Can you work these out from the model? Positions are in its coordinate system, mm. A direction names the side the tool comes from. Round coordinates to 2 decimals unless told otherwise and drop trailing zeros. Loops run counter-clockwise (first coordinate to the right, second up) from the corner with the lowest first, then second, coordinate; pieces in that order, holes last. Notation, with made-up numbers: (6.5, -39.75) -> (22.5, -39.75) arc R8 ccw to (22.5, -34.75) -> close; hole circle Ø5 at (64.5, 8). An arc over 180 degrees is marked (long way). Answer as a JSON object with one key per item and string values.
```python
from build123d import *

# Parameters (mm, degrees)
SKETCH1_W           = 45.23
SKETCH1_H           = 20.45
BOSS_EXTRUDE1_DEPTH = 1.6
SKETCH2_R           = 7.92
BOSS_EXTRUDE2_DEPTH = 12.2
BOSS_EXTRUDE3_DEPTH = 3.3
SKETCH4_W           = 4
SKETCH4_H           = 10.1
SKETCH4_W_2         = 8.68
SKETCH4_H_2         = 5.15
SKETCH4_W_3         = 10.3
SKETCH4_H_3         = 2.53
BOSS_EXTRUDE4_DEPTH = 1
SKETCH5_W           = 10.3
SKETCH5_H           = 2.53
BOSS_EXTRUDE5_DEPTH = 3.5
SKETCH6_R           = 0.25
BOSS_EXTRUDE6_DEPTH = 6.3
FILLET1_R           = 0.5
FILLET2_R           = 0.5
FILLET3_R           = 0.2
FILLET4_R           = 0.5
SKETCH7_R           = 0.55
CUT_EXTRUDE1_DEPTH  = 6.3


with BuildPart() as part:
    # Sketch1 → Boss-Extrude1 (new body)
    with BuildSketch(Plane(origin=(0, 0, 0), x_dir=(1, 0, 0), z_dir=(0, 1, 0))):
        with Locations((-22.615, 10.225)):
            Rectangle(SKETCH1_W, SKETCH1_H)
    extrude(amount=BOSS_EXTRUDE1_DEPTH)

    # Sketch2 → Boss-Extrude2 (add)
    with BuildSketch(Plane(origin=(0, 1.6, 0), x_dir=(1, 0, 0), z_dir=(0, 1, 0))):
        with Locations(Location((-35.515, 10.225, 0), (0, 0, 270))):
            Circle(SKETCH2_R)
        with Locations(Location((-9.715, 10.225, 0), (0, 0, 270))):
            Circle(SKETCH2_R)
    extrude(amount=BOSS_EXTRUDE2_DEPTH)

    # Sketch3 → Boss-Extrude3 (add)
    with BuildSketch(Plane(origin=(0, 1.6, 0), x_dir=(1, 0, 0), z_dir=(0, 1, 0))):
        with BuildLine():
            Line((-25.77, 19.5), (-19.46, 19.5))
            ThreePointArc((-19.46, 19.5), (-17.74, 17.78), (-19.46, 16.06))
            Line((-19.46, 16.06), (-25.77, 16.06))
            ThreePointArc((-25.77, 16.06), (-27.49, 17.78), (-25.77, 19.5))
        make_face()
    extrude(amount=BOSS_EXTRUDE3_DEPTH)

    # Sketch4 → Boss-Extrude4 (add)
    with BuildSketch(Plane.XZ):
        with Locations((-40.73, -10.225)):
            Rectangle(SKETCH4_W, SKETCH4_H)
        with Locations((-22.615, -10.225)):
            Rectangle(SKETCH4_W_2, SKETCH4_H_2)
        with Locations((-4.34, -10.225)):
            Rectangle(SKETCH4_W_2, SKETCH4_H_2)
        with Locations((-22.615, -1.465)):
            Rectangle(SKETCH4_W_3, SKETCH4_H_3)
    extrude(amount=BOSS_EXTRUDE4_DEPTH)

    # Sketch5 → Boss-Extrude5 (add)
    with BuildSketch(Plane.XZ.offset(1)):
        with Locations((-22.615, -1.465)):
            Rectangle(SKETCH5_W, SKETCH5_H)
    extrude(amount=BOSS_EXTRUDE5_DEPTH)

    # Sketch6 → Boss-Extrude6 (add)
    with BuildSketch(Plane.XY.offset(-0.2)):
        with Locations((-21.334010663, -4.5)):
            Circle(SKETCH6_R)
        with Locations((-18.759010663, -4.5)):
            Circle(SKETCH6_R)
        with Locations(Location((-23.895989337, -4.5, 0), (0, 0, 180))):
            Circle(SKETCH6_R)
        with Locations(Location((-26.470989337, -4.5, 0), (0, 0, 180))):
            Circle(SKETCH6_R)
    extrude(amount=BOSS_EXTRUDE6_DEPTH)

    # Fillet1
    # the kernel refuses this fillet: 0.5 mm, written as the material it adds along each edge
    with BuildSketch(Plane(origin=(-24.970989337, -4.5, -0.2), x_dir=(0, 0, -1), z_dir=(-1, 0, 0))) as fillet1_piece_1_section:
        with BuildLine():
            CenterArc((FILLET1_R, FILLET1_R), FILLET1_R, 180, 90)
            Line((0, FILLET1_R), (0, 0))
            Line((0, 0), (FILLET1_R, 0))
        make_face()
    fillet1_piece_1 = extrude(amount=3, mode=Mode.PRIVATE)
    fillet1_piece_1 = fillet1_piece_1 & Plane(origin=(-26.470989337, -4.5, -0.330121351), x_dir=(-1, 0, 0), z_dir=(0, 0, -1)) * Cylinder(0.25, 8, mode=Mode.PRIVATE)
    add(fillet1_piece_1)
    with BuildSketch(Plane(origin=(-22.395989337, -4.5, -0.2), x_dir=(0, 0, -1), z_dir=(-1, 0, 0))) as fillet1_piece_2_section:
        with BuildLine():
            CenterArc((FILLET1_R, FILLET1_R), FILLET1_R, 180, 90)
            Line((0, FILLET1_R), (0, 0))
            Line((0, 0), (FILLET1_R, 0))
        make_face()
    fillet1_piece_2 = extrude(amount=3, mode=Mode.PRIVATE)
    fillet1_piece_2 = fillet1_piece_2 & Plane(origin=(-23.895989337, -4.5, -0.330121351), x_dir=(-1, 0, 0), z_dir=(0, 0, -1)) * Cylinder(0.25, 8, mode=Mode.PRIVATE)
    add(fillet1_piece_2)
    with BuildSketch(Plane(origin=(-19.834010663, -4.5, -0.2), x_dir=(0, 0, -1), z_dir=(-1, 0, 0))) as fillet1_piece_3_section:
        with BuildLine():
            CenterArc((FILLET1_R, FILLET1_R), FILLET1_R, 180, 90)
            Line((0, FILLET1_R), (0, 0))
            Line((0, 0), (FILLET1_R, 0))
        make_face()
    fillet1_piece_3 = extrude(amount=3, mode=Mode.PRIVATE)
    fillet1_piece_3 = fillet1_piece_3 & Plane(origin=(-21.334010663, -4.5, -0.330121598), x_dir=(1, 0, 0), z_dir=(0, 0, -1)) * Cylinder(0.25, 8, mode=Mode.PRIVATE)
    add(fillet1_piece_3)
    with BuildSketch(Plane(origin=(-17.259010663, -4.5, -0.2), x_dir=(0, 0, -1), z_dir=(-1, 0, 0))) as fillet1_piece_4_section:
        with BuildLine():
            CenterArc((FILLET1_R, FILLET1_R), FILLET1_R, 180, 90)
            Line((0, FILLET1_R), (0, 0))
            Line((0, 0), (FILLET1_R, 0))
        make_face()
    fillet1_piece_4 = extrude(amount=3, mode=Mode.PRIVATE)
    fillet1_piece_4 = fillet1_piece_4 & Plane(origin=(-18.759010663, -4.5, -0.330121598), x_dir=(1, 0, 0), z_dir=(0, 0, -1)) * Cylinder(0.25, 8, mode=Mode.PRIVATE)
    add(fillet1_piece_4)

    # Fillet2
    fillet2_edges = [part.edges().sort_by_distance(p)[0] for p in [
        (-35.515, 13.8, -18.145),
        (-9.715, 13.8, -18.145),
    ]]
    fillet(fillet2_edges, radius=FILLET2_R)

    # Fillet3
    fillet3_edges = [part.edges().sort_by_distance(p)[0] for p in [
        (-27.49, 4.9, -17.78),
        (-22.615, 4.9, -16.06),
        (-17.74, 4.9, -17.78),
        (-22.615, 4.9, -19.5),
    ]]
    fillet(fillet3_edges, radius=FILLET3_R)

    # Fillet4
    fillet4_edges = [part.edges().sort_by_distance(p)[0] for p in [
        (-27.49, 1.6, -17.78),
        (-22.615, 1.6, -16.06),
        (-17.74, 1.6, -17.78),
        (-22.615, 1.6, -19.5),
    ]]
    fillet(fillet4_edges, radius=FILLET4_R)

    # Sketch7 → Cut-Extrude1 (cut)
    with BuildSketch(Plane(origin=(0, 1.6, 0), x_dir=(1, 0, 0), z_dir=(0, 1, 0))):
        with Locations(Location((-44.48, 19.7, 0), (0, 0, 270))):
            Circle(SKETCH7_R)
        with Locations(Location((-44.48, 0.75, 0), (0, 0, 270))):
            Circle(SKETCH7_R)
        with Locations(Location((-0.75, 0.75, 0), (0, 0, 270))):
            Circle(SKETCH7_R)
        with Locations(Location((-0.75, 19.7, 0), (0, 0, 270))):
            Circle(SKETCH7_R)
    extrude(amount=-CUT_EXTRUDE1_DEPTH, mode=Mode.SUBTRACT)


solid = part.part
```
Q1. I want a section at D-D, the plane x = -0.75. Write out the boundary of the cut face in (y, z).
Determined:
{"outline": "(-1, -12.8) -> (0, -12.8) -> (0, -19.15) -> (1.6, -19.15) -> (1.6, -1.3) -> (0, -1.3) -> (0, -7.65) -> (-1, -7.65) -> close; (0, -20.45) -> (1.6, -20.45) -> (1.6, -20.25) -> (0, -20.25) -> close; (0, -0.2) -> (1.6, -0.2) -> (1.6, 0) -> (0, 0) -> close"}
Q2. On a 3-axis mill with a long thin cutter (end or side, diameter ignored), from which of +Z, -Z, +X, -X, +Y, -Y can I reach the whole of each face in a straight line? I mean faces 4 (the flat face through (-22.7, -0.5, -7.65)), 5 (the flat face through (-23, -1, -10)), 6 (the cylindrical face through (-17.74, 3.38, -17.82)), 7 (the flat face through (-4.4, -0.5, -7.65)). Say none if no direction works.
Determined:
{"face 4": "+X, -Y", "face 5": "-Z, +X, -X, -Y", "face 6": "+Y", "face 7": "+Z, +X, -Y"}
Q3. I'm going to push flat-ended pins straight in: pin 1 (0.7 mm diameter, centred on x = -0.75, z = -19.7, fed in from +Y); pin 2 (10 mm diameter, centred on x = -12.5, z = -13.5, fed in from -Y); pin 3 (10 mm diameter, centred on x = -18, y = 6, fed in from +Z); pin 4 (1.4 mm diameter, centred on x = -0.75, z = -0.75, fed in from +Y). Where does each tip first touch, or does it pass through?
Determined:
{"pin 1": "through", "pin 2": "y = -1", "pin 3": "z = 0", "pin 4": "y = 1.6"}
Q4. We'd pull the mould along X, two halves only. Please class faces 1 (the flat face through (-27.765, -2, -1)), 2 (the flat face through (-23, -2, -2.73)), 3 (the cylindrical face through (-44.97, 0.81, -0.5)): pulls with the +X half, pulls with the -X half, needs draft (parallel to the pull), parting line crosses it, or undercut.
Determined:
{"face 1": "pulls with the -X half", "face 2": "needs draft", "face 3": "undercut"}
Q5. If I drill on L1, parallel to X at y = 1, z = -0.75; L2, parallel to Y at x = -38, z = -17; L3, parallel to X at y = 9, z = -11.5, over which ranges is the centre line in solid material (lowest first)? Write a range as [from, to].
Determined:
{"L1": "[-45.23, -45.03], [-43.93, -1.3], [-0.2, 0]", "L2": "[0, 13.8]", "L3": "[-43.33, -27.7], [-17.53, -1.9]"}
Q6. I want a section at C-C, the plane z = -1.75. Write out the boundary of the cut face in (x, y) (3 decimals), then the cut area to 3 significant figures.
Determined:
{"outline": "(-45.23, 0) -> (-27.765, 0) -> (-27.765, -4.5) -> (-17.465, -4.5) -> (-17.465, 0) -> (0, 0) -> (0, 1.6) -> (-45.23, 1.6) -> close", "area": "119 mm²"}
Q7. I want a section at B-B, the plane y = -0.5. Write out the boundary of the cut face in (x, z) (3 decimals).
Determined:
{"outline": "(-42.73, -15.275) -> (-38.73, -15.275) -> (-38.73, -5.175) -> (-42.73, -5.175) -> close; (-27.765, -2.73) -> (-17.465, -2.73) -> (-17.465, -0.2) -> (-27.765, -0.2) -> close; (-26.955, -12.8) -> (-18.275, -12.8) -> (-18.275, -7.65) -> (-26.955, -7.65) -> close; (-8.68, -12.8) -> (0, -12.8) -> (0, -7.65) -> (-8.68, -7.65) -> close"}
Q8. I want a section at A-A, the plane x = -44.48. Write out the boundary of the cut face in (y, z).
Determined:
{"outline": "(0, -20.45) -> (1.6, -20.45) -> (1.6, -20.25) -> (0, -20.25) -> close; (0, -19.15) -> (1.6, -19.15) -> (1.6, -1.3) -> (0, -1.3) -> close; (0, -0.2) -> (1.6, -0.2) -> (1.6, 0) -> (0, 0) -> close"}
